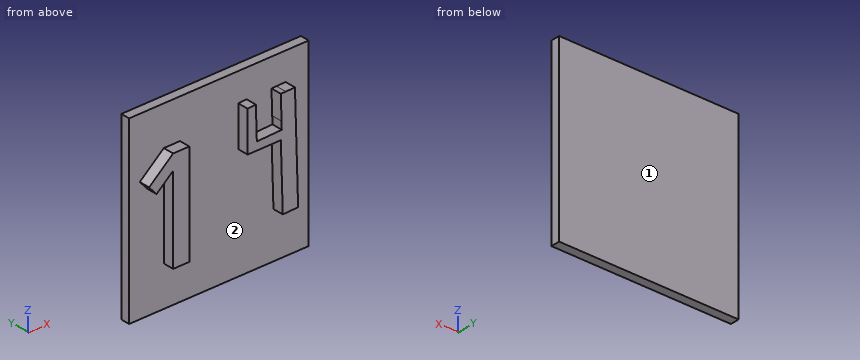
from build123d import *

# Parameters (mm, degrees)
F0_W     = 25.4
F0_H     = 25.4
F1_DEPTH = 1.27
F3_DEPTH = 1.524
F4_DEPTH = 1.524
F5_W     = 2.286
F5_H     = 1.560336
F6_DEPTH = 1.524


with BuildPart() as f1:
    # F0 (on Front) → F1 (new body)
    with BuildSketch(Plane.XZ):
        Rectangle(F0_W, F0_H)
    extrude(amount=F1_DEPTH)

    # F2 (on face) → F3 (join)
    with BuildSketch(Plane.XZ.offset(1.27)):
        Polygon((-10.138285, 3.041435), (-7.790129, 5.044031), (-7.790129, 7.174698), (-11.190262, 4.274936), align=None)
        Polygon((-7.790129, 5.044031), (-7.790129, -5.525302), (-5.504129, -5.525302), (-5.504129, 7.174698), (-7.790129, 7.174698), align=None)
    extrude(amount=F3_DEPTH)

    # F2 (on face) → F4 (join)
    with BuildSketch(Plane.XZ.offset(1.27)):
        Polygon((-7.790129, 5.044031), (-7.790129, -5.525302), (-5.504129, -5.525302), (-5.504129, 7.174698), (-7.790129, 7.174698), align=None)
        Polygon((-10.138285, 3.041435), (-7.790129, 5.044031), (-7.790129, 7.174698), (-11.190262, 4.274936), align=None)
        Polygon((3.909726, 8.777335), (2.750006, 8.712334), (2.750006, 3.041435), (7.441319, 3.041435), (7.719035, -6.231733), (9.88784, -6.166781), (9.439128, 8.816055), (8.14623, 8.777335), (7.441319, 8.777335), (7.543693, 5.358965), (7.576158, 4.274936), (4.04773, 4.169265), align=None)
    extrude(amount=F4_DEPTH)

    # F5 (on face) → F6 (join)
    with BuildSketch(Plane.XZ.offset(1.27)):
        with Locations((-6.647129, -6.30547)):
            Rectangle(F5_W, F5_H)
    extrude(amount=F6_DEPTH)


solid = f1.part
The model under review builds one solid part; all positions refer to its coordinate system, in mm. Face numbers are marked on the shaded views. Give positions to 0.01 mm unless a question says otherwise; leave off trailing zeros. Loops run counter-clockwise (first coordinate to the right, second up) from the corner with the lowest first, then second, coordinate; pieces in that order, holes last. Notation, with made-up numbers: (-1, 1) -> (44, 1) arc R19 cw to (44, 38) -> close; hole circle Ø10 at (77.25, 87). An arc over 180 degrees is marked (long way). Answer as a JSON object with one key per item and string values. Group by question number.
Q1. Take a section at C-C (x = 1.25). Write out the cut boundary in (y, z), plus the area to 3 significant figures.
Q2. Wall thickness on line 1 along X through (y, z) = (-2.1, 6); line 2 along Y through (x, z) = (11.5, 3.5); line 3 along X through (y, z) = (-1.65, 4.75): over which ranges is each line inside the solid? List them lowest first.
Q3. Draft analysis for pull direction X (two halves, no side actions). For the marked faces 1 and 2, state which applies: pulls with the +X half, pulls with the -X half, needs draft (parallel to the pull), parting line crosses it, or undercut.
Q4. Insertion check: pin 1 (1.2 mm diameter, centred on x = -7, y = -2, fed in from -Z); pin 2 (0.8 mm diameter, centred on y = -2.5, z = -1, fed in from +X); pin 3 (0.8 mm diameter, centred on y = -2, z = 0, fed in from -X). Each pin has a flat end and moves straight along its axis. Give the tip position at first contact, or say it passes through.
Q5. Take a section at B-B (z = -1.5). Write out the cut boundary in (x, y), plus the area to 4 significant figures.
Q6. Take a section at A-A (y = -1.6). Write out the cut boundary in (x, z), plus the area to 4 significant figures.
Q7. Take a section at D-D (z = 6.25). Write out the cut boundary in (x, y).
Answer below:
{
 "1": {"outline": "(-1.27, -12.7) -> (0, -12.7) -> (0, 12.7) -> (-1.27, 12.7) -> close", "area": "32.3 mm2"},
 "2": {"line 1": "x = -9.17 to -5.5, 2.75 to 3.99, 7.52 to 9.52", "line 2": "y = -1.27 to 0", "line 3": "x = -10.63 to -8.13, -7.79 to -5.5, 2.75 to 4.03, 7.56 to 9.56"},
 "3": {"face 1": "needs draft", "face 2": "undercut"},
 "4": {"pin 1": "stops at z = -7.09", "pin 2": "stops at x = 9.75", "pin 3": "stops at x = -7.79"},
 "5": {"outline": "(-12.7, -1.27) -> (-7.79, -1.27) -> (-7.79, -2.79) -> (-5.5, -2.79) -> (-5.5, -1.27) -> (7.58, -1.27) -> (7.58, -2.79) -> (9.75, -2.79) -> (9.75, -1.27) -> (12.7, -1.27) -> (12.7, 0) -> (-12.7, 0) -> close", "area": "39.05 mm2"},
 "6": {"outline": "(-11.19, 4.27) -> (-10.14, 3.04) -> (-7.79, 5.04) -> (-7.79, -7.09) -> (-5.5, -7.09) -> (-5.5, 7.17) -> (-7.79, 7.17) -> close; (2.75, 3.04) -> (7.44, 3.04) -> (7.72, -6.23) -> (9.89, -6.17) -> (9.44, 8.82) -> (8.15, 8.78) -> (7.44, 8.78) -> (7.54, 5.36) -> (7.58, 4.27) -> (4.05, 4.17) -> (3.91, 8.78) -> (2.75, 8.71) -> close", "area": "81.55 mm2"},
 "7": {"outline": "(-12.7, -1.27) -> (-8.87, -1.27) -> (-8.87, -2.79) -> (-5.5, -2.79) -> (-5.5, -1.27) -> (2.75, -1.27) -> (2.75, -2.79) -> (3.99, -2.79) -> (3.99, -1.27) -> (7.52, -1.27) -> (7.52, -2.79) -> (9.52, -2.79) -> (9.52, -1.27) -> (12.7, -1.27) -> (12.7, 0) -> (-12.7, 0) -> close"}
}
